CAD build for the part. Positions are in the model's coordinates, mm. Face numbers are marked on the shaded views. A direction names the side the tool comes from. Coordinates: 2 decimals unless noted, no trailing zeros. Order: outer loops, then holes, each group sorted by start corner. A loop starts at its lowest first (then second) coordinate and runs counter-clockwise, first axis right, second up. Notation, with made-up numbers: (69.25, 20.25) - (98.25, 20.25) arc R5 ccw to (98.25, 24.25) - close; hole circle Ø7 at (57, 18.25). An arc over 180 degrees is marked (long way). Use one line per item in the form item = value.
```python
from build123d import *

# Parameters (mm, degrees)
BOSS_EXTRUDE1_DEPTH = 25.5
SKETCH3_R           = 1.8
CUT_EXTRUDE1_DEPTH  = 4.5
SKETCH4_R           = 4
CUT_EXTRUDE2_DEPTH  = 2
SKETCH5_W           = 6
SKETCH5_H           = 25
CUT_EXTRUDE3_DEPTH  = 2
SKETCH6_R           = 2
CUT_EXTRUDE4_DEPTH  = 7
CUT_EXTRUDE5_START  = 7
SKETCH7_R           = 2
CUT_EXTRUDE5_DEPTH  = 7
SKETCH8_R           = 2
CUT_EXTRUDE6_DEPTH  = 7
CUT_EXTRUDE7_START  = 7
SKETCH9_R           = 2
CUT_EXTRUDE7_DEPTH  = 7


with BuildPart() as part:
    # Sketch1 → Revolve1 (revolve)
    with BuildSketch(Plane.XY, mode=Mode.PRIVATE) as revolve1_sk:
        Polygon((0, 0), (0, 27.8), (30, 27.8), (30, 25.8), (4.5, 25.8), (4.5, 0), align=None)
    revolve(revolve1_sk.sketch.rotate(Axis((-10, 0, 0), (1, 0, 0)), 90), axis=Axis((-10, 0, 0), (1, 0, 0)))

    # Sketch2 → Boss-Extrude1 (add)
    with BuildSketch(Plane(origin=(4.5, 0, 0), x_dir=(0, 0, -1), z_dir=(1, 0, 0))):
        with BuildLine():
            Line((-4, 17.5), (4, 17.5))
            ThreePointArc((4, 17.5), (4.707106781, 17.792893219), (5, 18.5))
            Line((5, 18.5), (5, 26.5))
            ThreePointArc((5, 26.5), (4.707106781, 27.207106781), (4, 27.5))
            Line((4, 27.5), (-4, 27.5))
            ThreePointArc((-4, 27.5), (-4.707106781, 27.207106781), (-5, 26.5))
            Line((-5, 26.5), (-5, 18.5))
            ThreePointArc((-5, 18.5), (-4.707106781, 17.792893219), (-4, 17.5))
        make_face()
        with BuildLine():
            Line((-4, -27.5), (4, -27.5))
            ThreePointArc((4, -27.5), (4.707106781, -27.207106781), (5, -26.5))
            Line((5, -26.5), (5, -18.5))
            ThreePointArc((5, -18.5), (4.707106781, -17.792893219), (4, -17.5))
            Line((4, -17.5), (-4, -17.5))
            ThreePointArc((-4, -17.5), (-4.707106781, -17.792893219), (-5, -18.5))
            Line((-5, -18.5), (-5, -26.5))
            ThreePointArc((-5, -26.5), (-4.707106781, -27.207106781), (-4, -27.5))
        make_face()
        with BuildLine():
            Line((-26.5, -5), (-18.5, -5))
            ThreePointArc((-18.5, -5), (-17.792893219, -4.707106781), (-17.5, -4))
            Line((-17.5, -4), (-17.5, 4))
            ThreePointArc((-17.5, 4), (-17.792893219, 4.707106781), (-18.5, 5))
            Line((-18.5, 5), (-26.5, 5))
            ThreePointArc((-26.5, 5), (-27.207106781, 4.707106781), (-27.5, 4))
            Line((-27.5, 4), (-27.5, -4))
            ThreePointArc((-27.5, -4), (-27.207106781, -4.707106781), (-26.5, -5))
        make_face()
        with BuildLine():
            Line((18.5, -5), (26.5, -5))
            ThreePointArc((26.5, -5), (27.207106781, -4.707106781), (27.5, -4))
            Line((27.5, -4), (27.5, 4))
            ThreePointArc((27.5, 4), (27.207106781, 4.707106781), (26.5, 5))
            Line((26.5, 5), (18.5, 5))
            ThreePointArc((18.5, 5), (17.792893219, 4.707106781), (17.5, 4))
            Line((17.5, 4), (17.5, -4))
            ThreePointArc((17.5, -4), (17.792893219, -4.707106781), (18.5, -5))
        make_face()
    extrude(amount=BOSS_EXTRUDE1_DEPTH)

    # Sketch3 → Cut-Extrude1 (cut)
    with BuildSketch(Plane(origin=(0, 0, 0), x_dir=(0, 0, -1), z_dir=(1, 0, 0))):
        with Locations((-8.84, 8.84)):
            Circle(SKETCH3_R)
        with Locations((-8.84, -8.84)):
            Circle(SKETCH3_R)
        with Locations((8.84, 8.84)):
            Circle(SKETCH3_R)
        with Locations((8.84, -8.84)):
            Circle(SKETCH3_R)
    extrude(amount=CUT_EXTRUDE1_DEPTH, mode=Mode.SUBTRACT)

    # Sketch4 → Cut-Extrude2 (cut)
    with BuildSketch(Plane(origin=(0, 0, 0), x_dir=(0, 0, -1), z_dir=(1, 0, 0))):
        Circle(SKETCH4_R)
    extrude(amount=CUT_EXTRUDE2_DEPTH, mode=Mode.SUBTRACT)

    # Sketch5 → Cut-Extrude3 (cut)
    with BuildSketch(Plane(origin=(0, 0, 0), x_dir=(0, 0, -1), z_dir=(1, 0, 0))):
        with Locations((0, -15.5)):
            Rectangle(SKETCH5_W, SKETCH5_H)
    extrude(amount=CUT_EXTRUDE3_DEPTH, mode=Mode.SUBTRACT)

    # Sketch6 → Cut-Extrude4 (cut)
    with BuildSketch(Plane(origin=(0, 27.8, 0), x_dir=(1, 0, 0), z_dir=(0, 1, 0))):
        with Locations(Location((15, 0, 0), (0, 0, 270))):
            Circle(SKETCH6_R)
    extrude(amount=-CUT_EXTRUDE4_DEPTH, mode=Mode.SUBTRACT)

    # Sketch7 → Cut-Extrude5 (cut)
    with BuildSketch(Plane(origin=(0, -27.8, 0), x_dir=(1, 0, 0), z_dir=(0, 1, 0)).offset(CUT_EXTRUDE5_START)):
        with Locations(Location((15, 0, 0), (0, 0, 270))):
            Circle(SKETCH7_R)
    extrude(amount=-CUT_EXTRUDE5_DEPTH, mode=Mode.SUBTRACT)

    # Sketch8 → Cut-Extrude6 (cut)
    with BuildSketch(Plane.XY.offset(27.8)):
        with Locations((15, 0)):
            Circle(SKETCH8_R)
    extrude(amount=-CUT_EXTRUDE6_DEPTH, mode=Mode.SUBTRACT)

    # Sketch9 → Cut-Extrude7 (cut)
    with BuildSketch(Plane.XY.offset(-27.8).offset(CUT_EXTRUDE7_START)):
        with Locations((15, 0)):
            Circle(SKETCH9_R)
    extrude(amount=-CUT_EXTRUDE7_DEPTH, mode=Mode.SUBTRACT)


solid = part.part
```
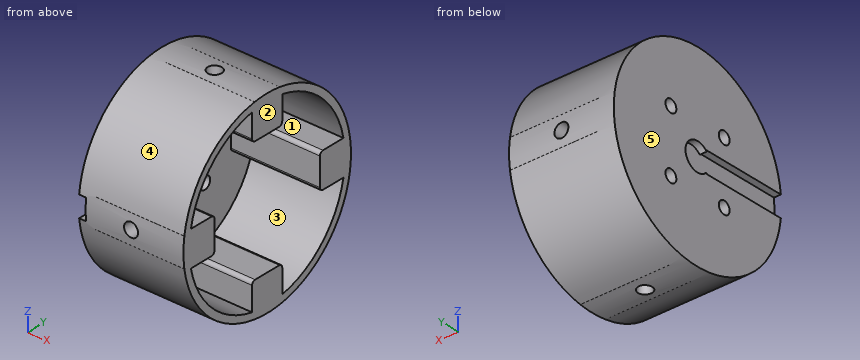
Item 1: Drill centre lines: line 1 (Z direction, x = 15, y = -23); line 2 (X direction, y = 0, z = -26.25); line 3 (Z direction, x = 1, y = 8). Where is each one in solid material? Low to high. Write a range as [from, to].
Derived:
line_1 = [-15.62, -11.69], [-5, -2], [2, 5], [11.69, 15.62]
line_2 = [0, 13], [17, 30]
line_3 = [-26.62, -10.43], [-7.25, 7.25], [10.43, 26.62]
Item 2: Cut at B-B, the plane y = 8.84. Write the cut outline in (x, z), plus the area to 3 significant figures.
Derived:
outline = (0, -26.36) - (30, -26.36) - (30, -24.24) - (4.5, -24.24) - (4.5, -10.64) - (0, -10.64) - close; (0, -7.04) - (4.5, -7.04) - (4.5, 7.04) - (0, 7.04) - close; (0, 10.64) - (4.5, 10.64) - (4.5, 24.24) - (30, 24.24) - (30, 26.36) - (0, 26.36) - close
area = 313 mm²
Item 3: Cut at D-D, the plane z = -21.5. Write the cut outline in (x, y).
Derived:
outline = (0, -17.62) - (30, -17.62) - (30, -14.26) - (4.5, -14.26) - (4.5, -5) - (30, -5) - (30, 5) - (4.5, 5) - (4.5, 14.26) - (30, 14.26) - (30, 17.62) - (0, 17.62) - close; hole circle Ø4 at (15, 0)
Item 4: 3-axis set-ups, long thin cutter, end or side, ignore diameter. For the marked faces 1 and 2: which of +Z, -Z, +X, -X, +Y, -Y reach the whole face in a straight line?
Derived:
face_1 = +X
face_2 = +Z, -Z, +X, +Y, -Y
Item 5: Two-plate mould, pull along Y, no slides. Class the marked faces 3, 4 and 5: +Y half, -Y half, draft (parallel to the pull), parting line (faces both ways), or undercut.
Derived:
face_3 = undercut
face_4 = parting line
face_5 = draft
Item 6: Cut at C-C, the plane z = 0. Write the cut outline in (x, y).
Derived:
outline = (0, 4) - (2, 4) - (2, -27.8) - (13, -27.8) - (13, -20.8) - (17, -20.8) - (17, -27.8) - (30, -27.8) - (30, -17.5) - (4.5, -17.5) - (4.5, 17.5) - (30, 17.5) - (30, 27.8) - (17, 27.8) - (17, 20.8) - (13, 20.8) - (13, 27.8) - (0, 27.8) - close
Item 7: Cut at A-A, the plane z = 8.5. Write the cut outline in (x, y).
Derived:
outline = (0, -26.47) - (30, -26.47) - (30, -24.36) - (4.5, -24.36) - (4.5, -10.61) - (0, -10.61) - close; (0, -7.07) - (4.5, -7.07) - (4.5, 7.07) - (0, 7.07) - close; (0, 10.61) - (4.5, 10.61) - (4.5, 24.36) - (30, 24.36) - (30, 26.47) - (0, 26.47) - close
Item 8: Drop flat-ended pins along their axis: pin 1 (6 mm diameter, centred on x = 6.5, z = 7.5, fed in from -Y); pin 2 (2 mm diameter, centred on x = 19.5, z = -23.5, fed in from -Y); pin 3 (3 mm diameter, centred on y = -15.5, z = 17, fed in from +X). Give the stop position or say it passes through.
Derived:
pin_1 = -27.43
pin_2 = -16.33
pin_3 = 4.5
